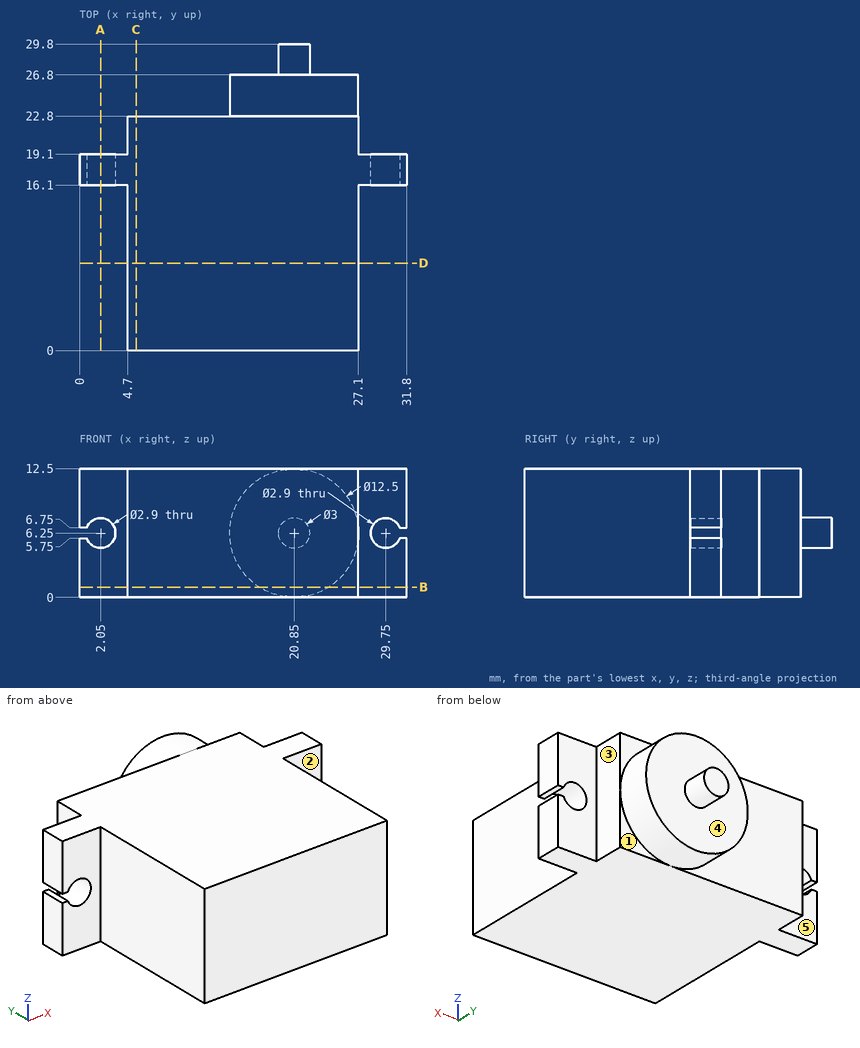
Answer from the drawing. Dimensions are ordinates in mm from the lowest x, y and z of the part. A direction names the side the tool comes from. Coordinates: 2 decimals unless noted, no trailing zeros. Order: outer loops, then holes, each group sorted by start corner. A loop starts at its lowest first (then second) coordinate and runs counter-clockwise, first axis right, second up. Notation, with made-up numbers: M 20.25,53 L 26.25,53 A12 cw 26.25,61 Z; hole C -5,-13.75 d8. An arc over 180 degrees is marked long. Put each result on its own line as item: value. Start each with the question number.
Item 1: Given pin 1 Ø5 at (x, z) = (1.5, 8.5) entering from +Y; pin 2 Ø1.9 at (y, z) = (20, 9) entering from -X; pin 3 Ø5 at (x, z) = (28.5, 4.5) entering from +Y; pin 4 Ø1.5 at (x, y) = (13, 26.5) entering from -Z, each flat-ended and moving along its own axis, determine where each tip first touches the part or whether it passes through.
Item 2: Section A-A, the plane x = 2.05 is taken. Determine the outline of the cut face in (y, z), plus the area to 3 significant figures.
Item 3: Section C-C, the plane x = 5.5 is taken. Determine the outline of the cut face in (y, z).
Item 4: For the marked faces 1, 2, 3, 4 and 5, determine the directions among +Z, -Z, +X, -X, +Y, -Y from which every point of the face is accessible in a straight line to the end or side of a thin tool.
Item 5: Consider probe 1 along Z at (x, y) = (2.05, 17.25); probe 2 along X at (y, z) = (13, 1); probe 3 along Y at (x, z) = (28, 11.25). Determine where each line is inside the solid, lowest interval first. Write a range as [from, to].
Item 6: Section D-D, the plane y = 8.5 is taken. Determine the outline of the cut face in (x, z), plus the area to 3 significant figures.
Item 7: Section B-B, the plane z = 1 is taken. Determine the outline of the cut face in (x, y), plus the area to 3 significant figures.
Computed:
1. pin 1: stops at y = 19.1
1. pin 2: stops at x = 0
1. pin 3: stops at y = 26.8
1. pin 4: passes through
2. outline: M 16.1,0 L 19.1,0 L 19.1,4.8 L 16.1,4.8 Z; M 16.1,7.7 L 19.1,7.7 L 19.1,12.5 L 16.1,12.5 Z
2. area: 28.8 mm2
3. outline: M 0,0 L 22.8,0 L 22.8,12.5 L 0,12.5 Z
4. face 1: -Z, +X, +Y
4. face 2: +Z, -Z, +X, -Y
4. face 3: +Z, -Z, +X, +Y
4. face 4: +Y
4. face 5: +Z, -Z, -X, +Y
5. probe 1: z = [0, 4.8], [7.7, 12.5]
5. probe 2: x = [4.7, 27.1]
5. probe 3: y = [16.1, 19.1]
6. outline: M 4.7,0 L 27.1,0 L 27.1,12.5 L 4.7,12.5 Z
6. area: 280 mm2
7. outline: M 0,16.1 L 4.7,16.1 L 4.7,0 L 27.1,0 L 27.1,16.1 L 31.8,16.1 L 31.8,19.1 L 27.1,19.1 L 27.1,22.8 L 24.24,22.8 L 24.24,26.8 L 17.46,26.8 L 17.46,22.8 L 4.7,22.8 L 4.7,19.1 L 0,19.1 Z
7. area: 566 mm2
